Check sheet for the drawn part. Datum: minimum x, y, z corner. Units: mm. Coordinates: 2 decimals unless noted, no trailing zeros. Write each loop counter-clockwise with the first axis right and the second up, starting at its lowest first coordinate (ties: lowest second). Pieces come first, ordered by that corner, then holes. Notation, with made-up numbers: (75, 42) -> (118, 42) arc R16 cw to (118, 72) -> close; hole circle Ø7 at (-34.5, 11.25). An arc over 180 degrees is marked (long way). Write item = value, one per line. Start each with the question number.
(1) Section check C-C (x = 15). Record the cut outline in (y, z).
(2) Section check D-D (y = 0.55). Record the cut outline in (x, z), plus the area to 3 significant figures.
(3) Section check B-B (z = 29). Record the cut outline in (x, y), plus the area to 3 significant figures.
(4) Section check A-A (z = 52.5). Record the cut outline in (x, y).
(5) Material ranges on probe 1 along Z at (x, y) = (52.5, 2.7); probe 2 along X at (y, z) = (2.1, 29), recorded low to high. Write a range as [from, to].
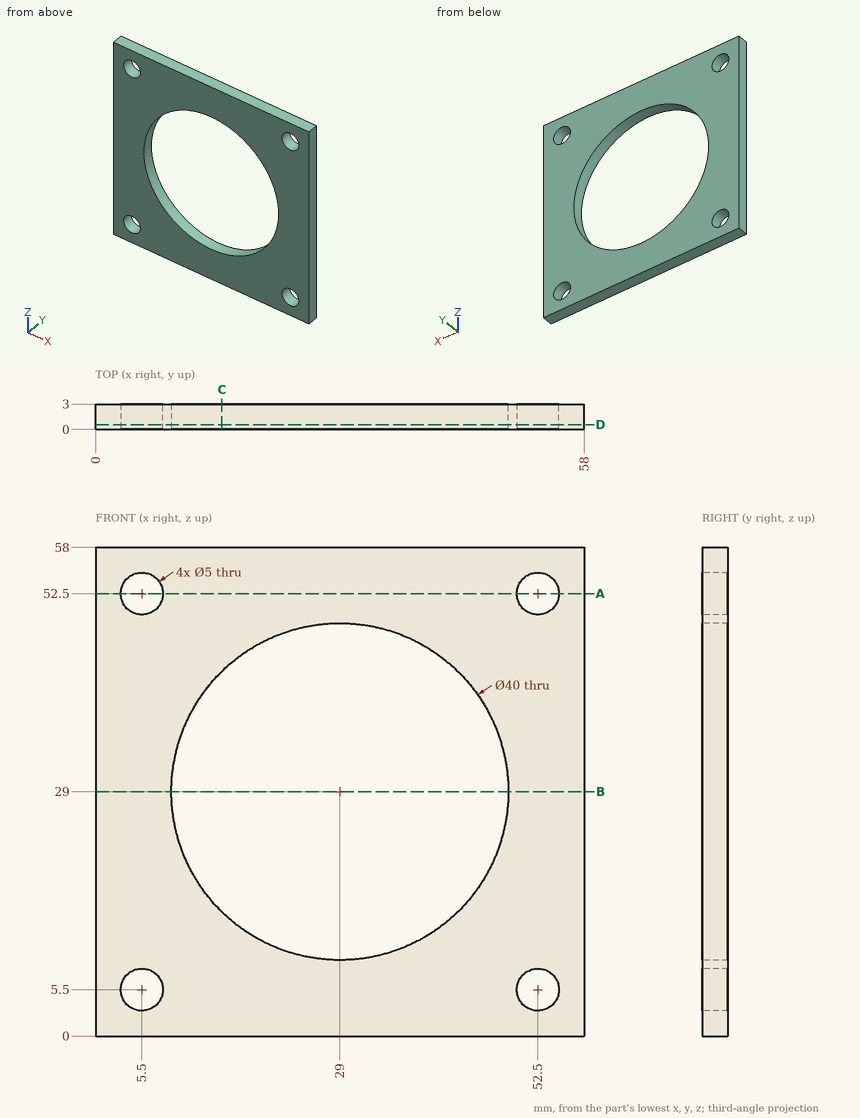
Response:
q1.outline = (0, 0) -> (3, 0) -> (3, 14.72) -> (0, 14.72) -> close; (0, 43.28) -> (3, 43.28) -> (3, 58) -> (0, 58) -> close
q2.outline = (0, 0) -> (58, 0) -> (58, 58) -> (0, 58) -> close; hole circle Ø5 at (5.5, 5.5); hole circle Ø5 at (5.5, 52.5); hole circle Ø40 at (29, 29); hole circle Ø5 at (52.5, 5.5); hole circle Ø5 at (52.5, 52.5)
q2.area = 2,030 mm2
q3.outline = (0, 0) -> (9, 0) -> (9, 3) -> (0, 3) -> close; (49, 0) -> (58, 0) -> (58, 3) -> (49, 3) -> close
q3.area = 54.0 mm2
q4.outline = (0, 0) -> (3, 0) -> (3, 3) -> (0, 3) -> close; (8, 0) -> (50, 0) -> (50, 3) -> (8, 3) -> close; (55, 0) -> (58, 0) -> (58, 3) -> (55, 3) -> close
q5.probe_1 = [0, 3], [8, 50], [55, 58]
q5.probe_2 = [0, 9], [49, 58]
